```python
from build123d import *

# Parameters (mm, degrees)
SKETCH_R        = 6.5
PAD_DEPTH       = 6
SKETCH001_R     = 1.75
POCKET_DEPTH    = 25.501
SKETCH002_R     = 2.9
POCKET001_DEPTH = 19.501


with BuildPart() as part:
    # Sketch → Pad (new body)
    with BuildSketch(Plane.XY):
        with BuildLine():
            ThreePointArc((9.5, 16), (0, 25.5), (-9.5, 16))
            ThreePointArc((-20, 5), (-12.546382, 8.396547), (-9.5, 16))
            Line((-20, 0), (-20, 5))
            Line((-20, 0), (20, 0))
            Line((20, 0), (20, 5))
            ThreePointArc((9.5, 16), (12.546382, 8.396547), (20, 5))
        make_face()
        with Locations((0, 16)):
            Circle(SKETCH_R, mode=Mode.SUBTRACT)
    extrude(amount=PAD_DEPTH)

    # Sketch001 (on Face4 of Pad) → Pocket (cut, through all)
    with BuildSketch(Plane.XZ):
        with Locations((-12, 3)):
            Circle(SKETCH001_R)
        with Locations((12, 3)):
            Circle(SKETCH001_R)
    extrude(amount=-POCKET_DEPTH, mode=Mode.SUBTRACT)

    # Sketch002 (on Face4 of Pad) → Pocket001 (cut, through all)
    with BuildSketch(Plane.XZ.offset(-6)):
        with Locations((-12, 3)):
            Circle(SKETCH002_R)
        with Locations((12, 3)):
            Circle(SKETCH002_R)
    extrude(amount=-POCKET001_DEPTH, mode=Mode.SUBTRACT)


solid = part.part
```
Can you work these out from the model? Positions are in its coordinate system, mm. A direction names the side the tool comes from. Round coordinates to 2 decimals unless told otherwise and drop trailing zeros. Loops run counter-clockwise (first coordinate to the right, second up) from the corner with the lowest first, then second, coordinate; pieces in that order, holes last. Notation, with made-up numbers: M 26.25,67.25 L 61.25,67.25 A23 ccw 61.25,77.25 Z; hole C 22,81.25 d10. An arc over 180 degrees is marked long. Answer in a Markdown table with one row per item.
1. Thinking about a two-plate mould opening in X: for faces 3 (the face through (-20, 2, 3)), 4 (the face through (0, 0, 3)), 5 (the face through (15.421, 6.235, 2.958)), 6 (the face through (-9.234, 10.861, 3.871)), which applies, pulls with the +X half, pulls with the -X half, needs draft (parallel to the pull), parting line crosses it, or undercut?
Established:
| item | result |
|---|---|
| face 3 | pulls with the -X half |
| face 4 | needs draft |
| face 5 | pulls with the +X half |
| face 6 | undercut |
2. Please list where these lines run through material, in increasing order: line 1 (Y direction, x = 0, z = 2.15); line 2 (Z direction, x = -12, y = 2.35); line 3 (X direction, y = 15.75, z = 1.25). Write a range as from..to.
Established:
| item | result |
|---|---|
| line 1 | 0..9.5, 22.5..25.5 |
| line 2 | 0..1.25, 4.75..6 |
| line 3 | -9.5..-6.5, 6.5..9.5 |
3. If we section it at A-A, the plane x = 0: Please give me the cut outline in (y, z).
Established:
| item | result |
|---|---|
| outline | M 0,0 L 9.5,0 L 9.5,6 L 0,6 Z; M 22.5,0 L 25.5,0 L 25.5,6 L 22.5,6 Z |
4. If we section it at C-C, the plane y = 10.25: Please give me the cut outline in (x, z).
Established:
| item | result |
|---|---|
| outline | M -11.12,0 L -3.03,0 L -3.03,6 L -11.12,6 L -11.12,5.76 A2.9 cw -11.12,0.24 Z; M 3.03,0 L 11.12,0 L 11.12,0.24 A2.9 cw 11.12,5.76 L 11.12,6 L 3.03,6 Z |
5. If we section it at B-B, the plane z = 2: Please give me the cut outline in (x, y).
Established:
| item | result |
|---|---|
| outline | M -20,0 L -13.44,0 L -13.44,6 L -14.72,6 L -14.72,6.63 A11.01 cw -20,5 Z; M -10.56,0 L 10.56,0 L 10.56,6 L 9.28,6 L 9.28,18.04 A9.5 ccw -9.28,18.04 L -9.28,6 L -10.56,6 Z; M 13.44,0 L 20,0 L 20,5 A11.01 cw 14.72,6.63 L 14.72,6 L 13.44,6 Z; hole C 0,16 d13 |
6. I'm going to push flat-ended pins straight in: pin 1 Ø2 at (y, z) = (14.5, 0.5) entering from -X; pin 2 Ø1.7 at (x, z) = (-13, 3) entering from +Y. Where does each tip first touch, or does it pass through?
Established:
| item | result |
|---|---|
| pin 1 | x = -9.79 |
| pin 2 | y = 6 |
7. If we section it at D-D, the plane y = 7: Please give me the cut outline in (x, z), plus the area to 3 significant figures.
Established:
| item | result |
|---|---|
| outline | M -14.17,0 L 14.17,0 L 14.17,1.07 A2.9 cw long 14.17,4.93 L 14.17,6 L -14.17,6 L -14.17,4.93 A2.9 cw long -14.17,1.07 Z |
| area | 121 mm² |
8. On a 3-axis mill with a long thin cutter (end or side, diameter ignored), from which of +Z, -Z, +X, -X, +Y, -Y can I reach the whole of each face in a straight line? I mean faces 1 (the face through (9.1, 10, 3)), 2 (the face through (0.209, 25.498, 2.958)). Say none if no direction works.
Established:
| item | result |
|---|---|
| face 1 | +Y |
| face 2 | +Z, -Z, +Y |
